Here's how the part is built. I have some questions about the finished solid (model axes, mm). A direction names the side the tool comes from. Round coordinates to 2 decimals unless told otherwise and drop trailing zeros. Order: outer loops, then holes, each group sorted by start corner. A loop starts at its lowest first (then second) coordinate and runs counter-clockwise, first axis right, second up. Notation, with made-up numbers: (49.5, 55.25) -> (92.5, 55.25) arc R15 ccw to (92.5, 72.25) -> close; hole circle Ø11 at (-25, 50.5). An arc over 180 degrees is marked (long way). One line per item, written item: value.
```python
from build123d import *

# Parameters (mm, degrees)
F0_W     = 200
F0_H     = 137.5
F1_DEPTH = 37.45
F2_W     = 200
F2_H     = 20
F3_DEPTH = 15
F4_W     = 30
F4_H     = 5
F5_DEPTH = 35
F7_DEPTH = 15
F9_DEPTH = 7.6


with BuildPart() as f1:
    # F0 (on Top) → F1 (new body)
    with BuildSketch(Plane.XY):
        Rectangle(F0_W, F0_H)
    extrude(amount=F1_DEPTH)

    # F2 (on face) → F3 (cut)
    with BuildSketch(Plane.XY.offset(37.45)):
        Rectangle(F2_W, F2_H)
    extrude(amount=-F3_DEPTH, mode=Mode.SUBTRACT)

    # F4 (on face) → F5 (cut)
    with BuildSketch(Plane.XY.offset(37.45)):
        Polygon((11.49270311, 10), (-11.49270311, 10), (-15, 10), (-15, -10), (15, -10), (15, 10), align=None)
        with Locations((0, -12.5)):
            Rectangle(F4_W, F4_H)
    extrude(amount=-F5_DEPTH, mode=Mode.SUBTRACT)

    # F6 (on Right) → F7 (cut, symmetric)
    with BuildSketch(Plane.YZ):
        Polygon((10, 37.45), (10, 2.45), (27.9449588614, 35.45), (29.0325321257, 37.45), align=None)
        Polygon((29.0325321257, 37.45), (27.9449588614, 35.45), (68.75, 35.45), (68.75, 37.45), align=None)
    extrude(amount=F7_DEPTH, both=True, mode=Mode.SUBTRACT)

    # F8 (on face) → F9 (cut)
    with BuildSketch(Plane.XY.offset(37.45)):
        with BuildLine():
            Line((76.5, -52.875), (100, -52.875))
            Line((100, -52.875), (100, -25.875))
            Line((100, -25.875), (76.5, -25.875))
            ThreePointArc((76.5, -25.875), (75.4748737342, -28.3498737342), (73, -29.375))
            Line((73, -29.375), (73, -49.375))
            ThreePointArc((73, -49.375), (75.4748737342, -50.4001262658), (76.5, -52.875))
        make_face()
        with BuildLine():
            ThreePointArc((73, -49.375), (70.5251262658, -55.3498737342), (76.5, -52.875))
            Line((76.5, -52.875), (73, -52.875))
            Line((73, -52.875), (73, -49.375))
        make_face()
        with BuildLine():
            Line((73, -52.875), (76.5, -52.875))
            ThreePointArc((76.5, -52.875), (75.4748737342, -50.4001262658), (73, -49.375))
            Line((73, -49.375), (73, -52.875))
        make_face()
        with BuildLine():
            ThreePointArc((73, -29.375), (75.4748737342, -28.3498737342), (76.5, -25.875))
            Line((76.5, -25.875), (73, -25.875))
            Line((73, -25.875), (73, -29.375))
        make_face()
        with BuildLine():
            Line((73, -25.875), (76.5, -25.875))
            ThreePointArc((76.5, -25.875), (70.5251262658, -23.4001262658), (73, -29.375))
            Line((73, -29.375), (73, -25.875))
        make_face()
    extrude(amount=-F9_DEPTH, mode=Mode.SUBTRACT)


solid = f1.part
```
Q1. For P1, Ø24, axis at x = -6.5, y = 47, coming from the +Z side; P2, Ø12.5, axis at x = -1, y = 2, coming from the +Z side; P3, Ø2.5, axis at y = -39, z = 34, coming from the +X side, each with a flat end and sliding along its axis, tell me the tip position at first contact or that it passes through.
Answers:
P1: z = 37.45
P2: z = 2.45
P3: x = 73
Q2. I want a section at A-A on x = -88. Write out the boundary of the cut face in (y, z), then the cut area to 3 significant figures.
Answers:
outline: (-68.75, 0) -> (68.75, 0) -> (68.75, 37.45) -> (10, 37.45) -> (10, 22.45) -> (-10, 22.45) -> (-10, 37.45) -> (-68.75, 37.45) -> close
area: 4,850 mm2
Q3. I want a section at D-D on z = 10. Write out the boundary of the cut face in (x, y), then the cut area to 3 significant figures.
Answers:
outline: (-100, -68.75) -> (100, -68.75) -> (100, 68.75) -> (-100, 68.75) -> close; hole (-15, -15) -> (15, -15) -> (15, 14.11) -> (-15, 14.11) -> close
area: 26,600 mm2
Q4. I want a section at C-C on z = 32.5. Write out the boundary of the cut face in (x, y) (3 decimals), then the cut area to 3 significant figures.
Answers:
outline: (-100, -68.75) -> (100, -68.75) -> (100, -52.875) -> (76.5, -52.875) arc R3.5 cw (long way) to (73, -49.375) -> (73, -29.375) arc R3.5 cw (long way) to (76.5, -25.875) -> (100, -25.875) -> (100, -10) -> (15, -10) -> (15, -15) -> (-15, -15) -> (-15, -10) -> (-100, -10) -> close; (-100, 10) -> (-15, 10) -> (-15, 26.341) -> (15, 26.341) -> (15, 10) -> (100, 10) -> (100, 68.75) -> (-100, 68.75) -> close
area: 22,100 mm2
Q5. I need wall thicknesses on line 1 along Y through (x, z) = (46, 23.5); line 2 along X through (y, z) = (3, 22); line 3 along Z through (x, y) = (-39.5, 3). Which ranges of each line are inside material? Lowest first, please.
Answers:
line 1: -68.75 to -10, 10 to 68.75
line 2: -100 to -15, 15 to 100
line 3: 0 to 22.45
Q6. I want a section at B-B on y = 7. Write out the boundary of the cut face in (x, z), then the cut area to 3 significant figures.
Answers:
outline: (-100, 0) -> (100, 0) -> (100, 22.45) -> (15, 22.45) -> (15, 2.45) -> (-15, 2.45) -> (-15, 22.45) -> (-100, 22.45) -> close
area: 3,890 mm2
Q7. If we mould it in two halves opening along X, with no side actions, what happens to faces 6 (the face through (100, -1, 18)), 7 (the face through (-1, 1, 0)), 8 (the face through (-100, -1, 18)), 9 (the face through (-15, 8, 20))? For each: pulls with the +X half, pulls with the -X half, needs draft (parallel to the pull), parting line crosses it, or undercut.
Answers:
face 6: pulls with the +X half
face 7: needs draft
face 8: pulls with the -X half
face 9: undercut
Q8. Which directions (+Z, -Z, +X, -X, +Y, -Y) give clear straight access to the entire face, cutting with the end or side of a thin tool? Please do faces 1 (the face through (0, 48, 35.45)), 2 (the face through (57, 10, 30)), 3 (the face through (88, -25.875, 34)), 4 (the face through (-1, -68.75, 18)), 5 (the face through (70.61, -23.32, 33.7)).
Answers:
face 1: +Z, +Y
face 2: +Z, +X, -X
face 3: +Z, +X
face 4: +Z, -Z, +X, -X, -Y
face 5: +Z
